from build123d import *

# Parameters (mm, degrees)
F0_R     = 10.5045071993
F1_DEPTH = 20
F2_W     = 65.2672518045
F2_H     = 27.032835409
F3_DEPTH = 33.8
F5_DEPTH = 65.2672518045
F6_R     = 4.8229033698
F7_DEPTH = 121.2269564549
F9_DEPTH = 38.0423929


with BuildPart() as f1:
    # F0 (on Top) → F1 (new body)
    with BuildSketch(Plane.XY):
        with BuildLine():
            ThreePointArc((-77.745065093, 25), (-102.745065093, 0), (-77.745065093, -25))
            Line((-77.745065093, -25), (53.5661391914, -25))
            ThreePointArc((53.5661391914, -25), (78.5661391914, 0), (53.5661391914, 25))
            Line((53.5661391914, 25), (-77.745065093, 25))
        make_face()
        with Locations((-77.745065093, 0)):
            Circle(F0_R, mode=Mode.SUBTRACT)
        with BuildLine():
            ThreePointArc((64.4582820553, 0), (53.5661391914, -10.8921428639), (42.6739963275, 0))
            ThreePointArc((42.6739963275, 0), (53.5661391914, 10.8921428639), (64.4582820553, 0))
        make_face(mode=Mode.SUBTRACT)
    extrude(amount=F1_DEPTH)

    # F2 (on face) → F3 (join)
    with BuildSketch(Plane.XY.offset(20)):
        with Locations((-14.1527345404, -0.4750248045)):
            Rectangle(F2_W, F2_H)
    extrude(amount=F3_DEPTH)

    # F4 (on face) → F5 (join, through all)
    with BuildSketch(Plane.YZ.offset(18.4808913618)):
        with BuildLine():
            Line((-13.991442509, 53.8), (13.0413929, 53.8))
            ThreePointArc((13.0413929, 53.8), (-0.4750248045, 67.3164177045), (-13.991442509, 53.8))
        make_face()
    extrude(amount=-F5_DEPTH)

    # F6 (on face) → F7 (cut, through all)
    with BuildSketch(Plane.YZ.offset(18.4808913618)):
        with Locations((-0.4750248045, 53.8)):
            Circle(F6_R)
    extrude(amount=-F7_DEPTH, mode=Mode.SUBTRACT)

    # F8 (on face) → F9 (cut, through all)
    with BuildSketch(Plane(origin=(0, 13.0413929, 0), x_dir=(-1, 0, 0), z_dir=(0, 1, 0))):
        with BuildLine():
            Line((28.9868507534, 71.8440338969), (1.5166216763, 71.8440338969))
            Line((1.5166216763, 71.8440338969), (1.5166216763, 39.9625226855))
            ThreePointArc((1.5166216763, 39.9625226855), (15.2517362149, 26.227408147), (28.9868507534, 39.9625226855))
            Line((28.9868507534, 39.9625226855), (28.9868507534, 71.8440338969))
        make_face()
    extrude(amount=-F9_DEPTH, mode=Mode.SUBTRACT)


solid = f1.part
Read the model definition and answer for the solid it produces. Units are mm, in the model's axes. A direction names the side the tool comes from. Round coordinates to 2 decimals unless told otherwise and drop trailing zeros. Write each loop counter-clockwise with the first axis right and the second up, starting at its lowest first coordinate (ties: lowest second). Pieces come first, ordered by that corner, then holes.
1. Which of the six approach directions +Z, -Z, +X, -X, +Y, -Y give full straight-line access (tool end or side, diameter ignored) to faces 4 (the face through (-1.517, 0, 48)), 5 (the face through (-46.786, -1, 44)), 6 (the face through (-15, 13.041, 25)), 7 (the face through (18.481, -1, 44))?
2. Given pin 1 Ø12 at (y, z) = (13, 29) entering from -X; pin 2 Ø13.5 at (y, z) = (1, 56) entering from +X; pin 3 Ø5 at (x, y) = (-31.5, 8.5) entering from +Z, each flat-ended and moving along its own axis, determine where each tip first touches the part or whether it passes through.
3. The part is cut by section A-A, the plane z = 45. Determine the outline of the cut face in (x, y), then the cut area to 3 significant figures.
4. Determine the mould class of faces 1 (the face through (-37.762, -0.178, 67.313)), 2 (the face through (8.62, -1.52, 49.09)), 3 (the face through (-15, -13.991, 25)) for opening direction Y: pulls with the +Y half, pulls with the -Y half, needs draft (parallel to the pull), parting line crosses it, or undercut.
5. Straight lines are drawn through the part: L1, parallel to X at y = -9, z = 43.5; L2, parallel to Z at x = -70, y = 8; L3, parallel to X at y = 4.5, z = 25.5. For each, find the intervals that lie inside material, in ascending order.
6. The part is cut by section D-D, the plane x = -74. Determine the outline of the cut face in (y, z).
7. The part is cut by section C-C, the plane y = 0. Determine the outline of the cut face in (x, z).
Values:
1. face 4: +Z, +Y, -Y
1. face 5: +Z, -X, +Y, -Y
1. face 6: +Z, +X, -X, +Y
1. face 7: +Z, +X, +Y, -Y
2. pin 1: stops at x = -46.79
2. pin 2: stops at x = 18.48
2. pin 3: stops at z = 65.66
3. outline: (-46.79, -13.99) - (-28.99, -13.99) - (-28.99, 13.04) - (-46.79, 13.04) - close; (-1.52, -13.99) - (18.48, -13.99) - (18.48, 13.04) - (-1.52, 13.04) - close
3. area: 1,020 mm2
4. face 1: parting line crosses it
4. face 2: undercut
4. face 3: pulls with the -Y half
5. L1: x = -46.79 to -28.99, -1.52 to 18.48
5. L2: z = 0 to 20
5. L3: x = -46.79 to 18.48
6. outline: (-25, 0) - (-9.81, 0) - (-9.81, 20) - (-25, 20) - close; (9.81, 0) - (25, 0) - (25, 20) - (9.81, 20) - close
7. outline: (-102.75, 0) - (-88.25, 0) - (-88.25, 20) - (-102.75, 20) - close; (-67.24, 0) - (42.67, 0) - (42.67, 20) - (18.48, 20) - (18.48, 49) - (-1.52, 49) - (-1.52, 39.96) arc R13.74 cw to (-28.99, 39.96) - (-28.99, 49) - (-46.79, 49) - (-46.79, 20) - (-67.24, 20) - close; (-46.79, 58.6) - (-28.99, 58.6) - (-28.99, 67.31) - (-46.79, 67.31) - close; (-1.52, 58.6) - (18.48, 58.6) - (18.48, 67.31) - (-1.52, 67.31) - close; (64.46, 0) - (78.57, 0) - (78.57, 20) - (64.46, 20) - close
